Source: three-view drawing plus pictorial views. Frame: mm from the lowest corner of the part. A direction names the side the tool comes from. Give positions to 0.01 mm unless a question says otherwise; leave off trailing zeros. Loops run counter-clockwise (first coordinate to the right, second up) from the corner with the lowest first, then second, coordinate; pieces in that order, holes last. Notation, with made-up numbers: (52, -9.5) - (106, -9.5) arc R28 cw to (106, 14.5) - close; hole circle Ø6 at (-27, 78). An arc over 180 degrees is marked (long way). Answer as a JSON object with one key per item and string values. Group by question number.
(1) Section query A-A (x = 13). Return loops of the section in (y, z), plus the area to 3 significant figures.
(2) Material intervals for L1, parallel to Z at x = 14, y = 1.55; L2, parallel to Y at x = 16, z = 5.5; L3, parallel to Y at x = 6, z = 13, sorted ascending.
(3) Section query B-B (z = 10.25). Return loops of the section in (x, y).
(4) Access query for the marked faces 1, 2, 3 and 4. Directions: +Z, -Z, +X, -X, +Y, -Y. A direction counts if a zero-diameter tool reaches every point of the face in a straight line with its end or side. Return the directions, or none.
(5) Pin query (flat end, axial travel): P1, Ø0.5, axis at y = 1, z = 5.5, coming from the -X side; P2, Ø0.7, axis at y = 1, z = 23.5, coming from the +X side; P3, Ø11, axis at x = 24, z = 19, coming from the +Y side. Return the tip coordinate at first contact, or that it passes through.
(6) Mould query, pull axis X, two halves, no side actions, for the marked faces 5, 6 and 7. Classes: +X half, -X half, draft (parallel to the pull), parting line (faces both ways), or undercut.
(7) Section query C-C (y = 2.3). Return loops of the section in (x, z), plus the area to 3 significant figures.
(8) Section query D-D (x = 21.5). Return loops of the section in (y, z).
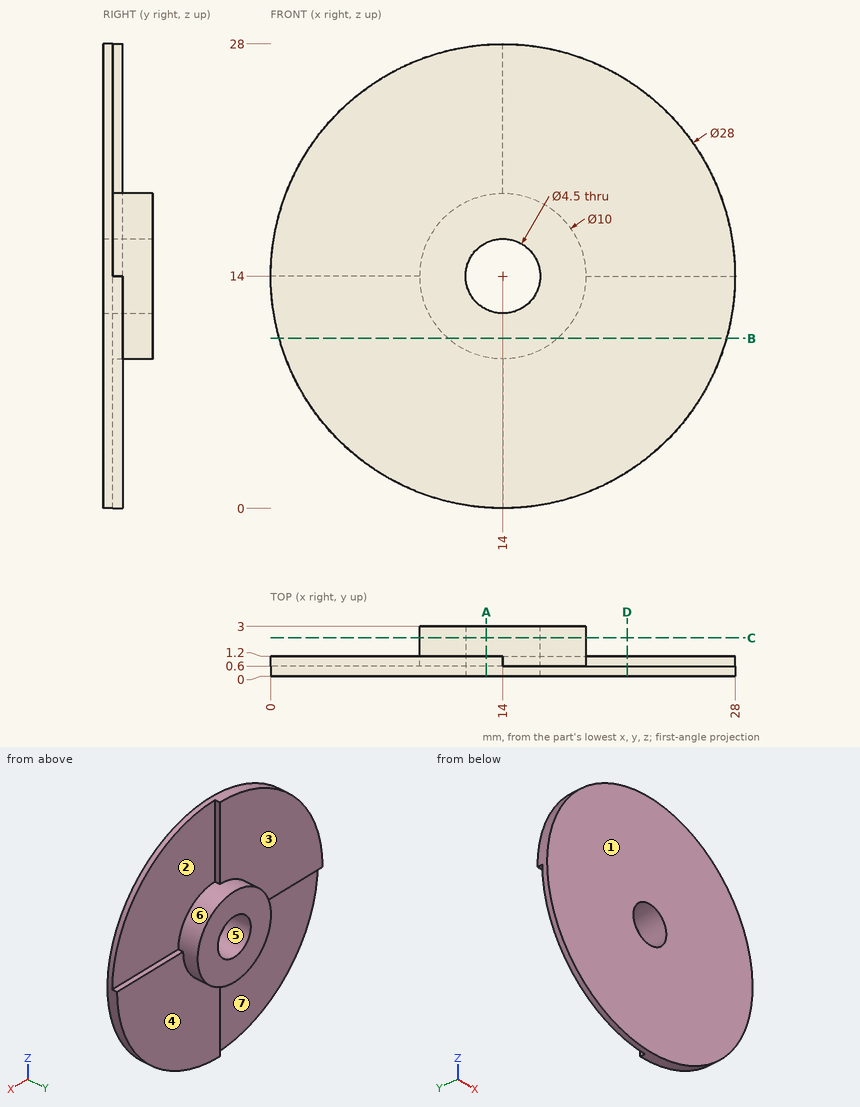
Recorded:
{
 "1": {"outline": "(0, 0.04) - (0.6, 0.04) - (0.6, 9.1) - (3, 9.1) - (3, 11.98) - (0, 11.98) - close; (0, 16.02) - (3, 16.02) - (3, 18.9) - (1.2, 18.9) - (1.2, 27.96) - (0, 27.96) - close", "area": "33.6 mm^2"},
 "2": {"L1": "z = 9 to 11.75, 16.25 to 19", "L2": "y = 0 to 1.2", "L3": "y = 0 to 0.6"},
 "3": {"outline": "(0.51, 0) - (27.49, 0) - (27.49, 1.2) - (17.31, 1.2) - (17.31, 3) - (10.69, 3) - (10.69, 0.6) - (0.51, 0.6) - close"},
 "4": {"face 1": "+Z, -Z, +X, -X, -Y", "face 2": "+Z, +X, +Y", "face 3": "+Z, -X, +Y", "face 4": "-Z, +X, +Y"},
 "5": {"P1": "stops at x = 14", "P2": "stops at x = 14", "P3": "stops at y = 1.2"},
 "6": {"face 5": "undercut", "face 6": "parting line", "face 7": "draft"},
 "7": {"outline": "circle Ø10 at (14, 14); hole circle Ø4.5 at (14, 14)", "area": "62.6 mm^2"},
 "8": {"outline": "(0, 2.18) - (1.2, 2.18) - (1.2, 14) - (0.6, 14) - (0.6, 25.82) - (0, 25.82) - close"}
}
